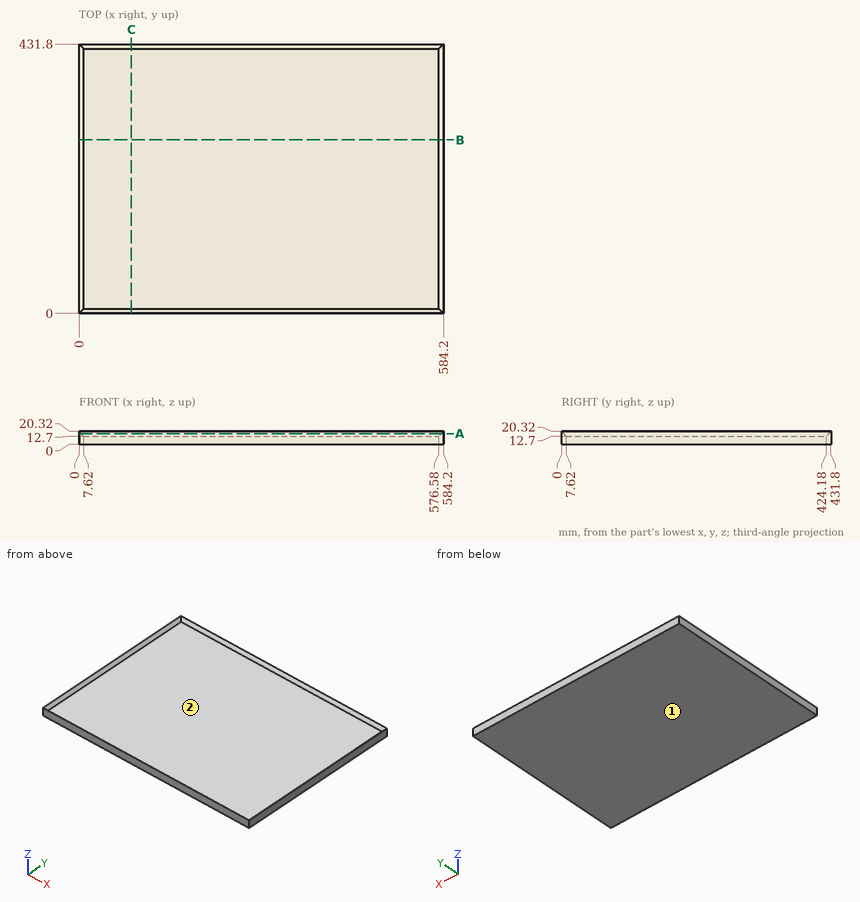
Print and shaded views of the part. All mm, measured from the part's lowest x, y and z. Round coordinates to 2 decimals unless told otherwise and drop trailing zeros. Order: outer loops, then holes, each group sorted by start corner. A loop starts at its lowest first (then second) coordinate and runs counter-clockwise, first axis right, second up.
Q1. Wall check: L1, parallel to Y at x = 386, z = 12.75; L2, parallel to Z at x = 414, y = 114.5; L3, parallel to Y at x = 214, z = 15. Give the ranges that are in metal, low to high.
Q2. Slice it at B-B (y = 278). Write the cut outline in (x, z).
Q3. Two-plate mould, pull along X, no slides. Class the marked faces 1 and 2: pulls with the +X half, pulls with the -X half, needs draft (parallel to the pull), parting line crosses it, or undercut.
Q4. Slice it at A-A (z = 17). Write the cut outline in (x, y), and give its area (3 significant figures).
Q5. Slice it at C-C (x = 84). Write the cut outline in (y, z), and give its area (3 significant figures).
Results below:
1. L1: y = 0 to 7.57, 424.23 to 431.8
1. L2: z = 0 to 12.7
1. L3: y = 0 to 5.32, 426.48 to 431.8
2. outline: (0, 0) - (584.2, 0) - (584.2, 20.32) - (576.58, 12.7) - (7.62, 12.7) - (0, 20.32) - close
3. face 1: needs draft
3. face 2: undercut
4. outline: (0, 0) - (584.2, 0) - (584.2, 431.8) - (0, 431.8) - close; hole (3.32, 3.32) - (580.88, 3.32) - (580.88, 428.48) - (3.32, 428.48) - close
4. area: 6,700 mm2
5. outline: (0, 0) - (431.8, 0) - (431.8, 20.32) - (424.18, 12.7) - (7.62, 12.7) - (0, 20.32) - close
5. area: 5,540 mm2
